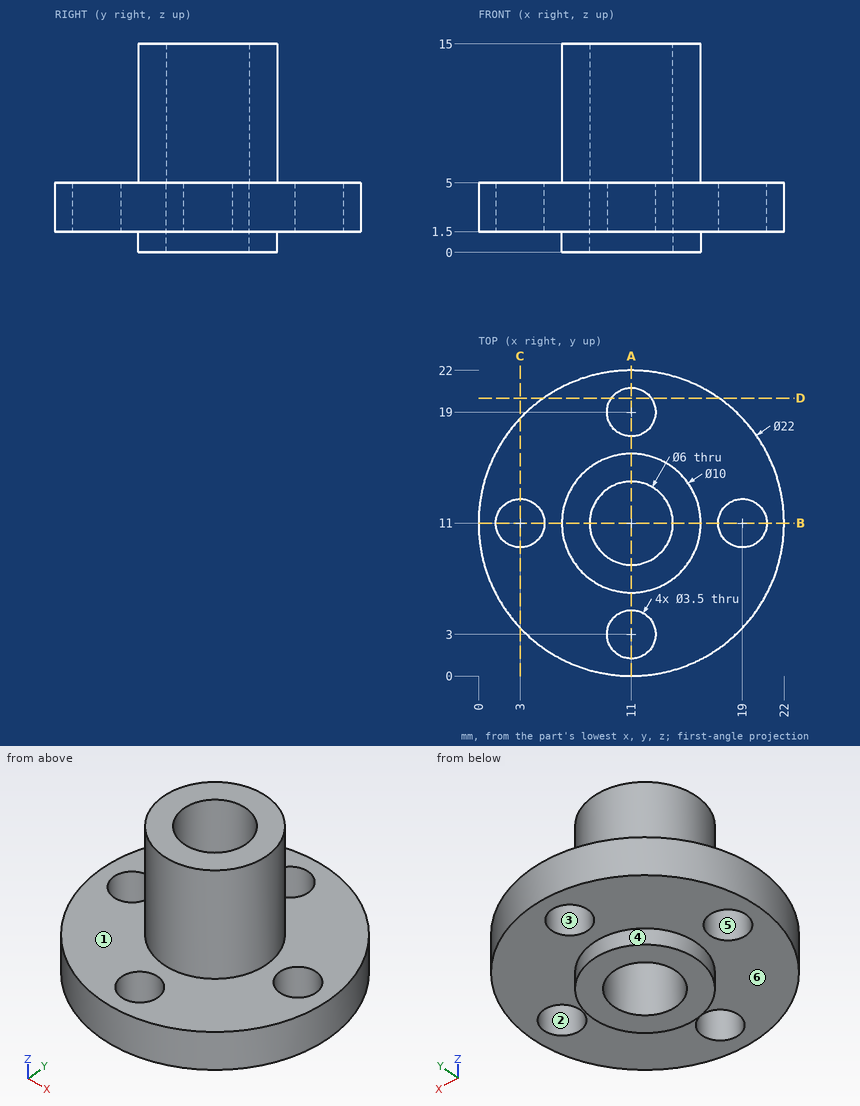
Source: three-view drawing plus pictorial views. Frame: mm from the lowest corner of the part. A direction names the side the tool comes from. Round coordinates to 2 decimals unless told otherwise and drop trailing zeros. Write each loop counter-clockwise with the first axis right and the second up, starting at its lowest first coordinate (ties: lowest second). Pieces come first, ordered by that corner, then holes. Notation, with made-up numbers: M 10,39.5 L 15,39.5 A11 cw 15,46.5 Z; hole C 19,-38.75 d7. An arc over 180 degrees is marked long. Write each question's results on one line, items separated by ' | '.
Q1. Access query for the marked faces 1 and 2. Directions: +Z, -Z, +X, -X, +Y, -Y. A direction counts if a zero-diameter tool reaches every point of the face in a straight line with its end or side. Return the directions, or none.
Results:
face 1: +Z | face 2: +Z, -Z
Q2. Section query A-A (x = 11). Return loops of the section in (y, z).
Results:
outline: M 0,1.5 L 1.25,1.5 L 1.25,5 L 0,5 Z; M 4.75,1.5 L 6,1.5 L 6,0 L 8,0 L 8,15 L 6,15 L 6,5 L 4.75,5 Z; M 14,0 L 16,0 L 16,1.5 L 17.25,1.5 L 17.25,5 L 16,5 L 16,15 L 14,15 Z; M 20.75,1.5 L 22,1.5 L 22,5 L 20.75,5 Z
Q3. Draft query along Y for the marked faces 3, 4, 5 and 6. Return one class per face: released by +Y, released by -Y, zero draft, split by the parting line, or undercut.
Results:
face 3: undercut | face 4: split by the parting line | face 5: undercut | face 6: zero draft
Q4. Section query D-D (y = 20). Return loops of the section in (x, z).
Results:
outline: M 4.68,1.5 L 9.56,1.5 L 9.56,5 L 4.68,5 Z; M 12.44,1.5 L 17.32,1.5 L 17.32,5 L 12.44,5 Z
Q5. Pin query (flat end, axial travel): P1, Ø1, axis at x = 15.5, z = 8, coming from the -Y side; P2, Ø3, axis at y = 8.5, z = 12, coming from the +X side; P3, Ø4, axis at x = 11, y = 19, coming from the +Z side. Return the tip coordinate at first contact, or that it passes through.
Results:
P1: stops at y = 8 | P2: stops at x = 15.9 | P3: stops at z = 5
Q6. Line query: line 1 along Y through (x, z) = (11, 3.45); line 2 along X through (y, z) = (9.5, 4.5); line 3 along Z through (x, y) = (17.25, 6.5). Output: solid intervals per line, ascending.
Results:
line 1: y = 0 to 1.25, 4.75 to 8, 14 to 17.25, 20.75 to 22 | line 2: x = 0.1 to 2.1, 3.9 to 8.4, 13.6 to 18.1, 19.9 to 21.9 | line 3: z = 1.5 to 5
Q7. Section query C-C (x = 3). Return loops of the section in (y, z).
Results:
outline: M 3.45,1.5 L 9.25,1.5 L 9.25,5 L 3.45,5 Z; M 12.75,1.5 L 18.55,1.5 L 18.55,5 L 12.75,5 Z
